Geometry check sheet. Reference: the model listing, model coordinates, mm. Face numbers are marked on the shaded views. A direction names the side the tool comes from. Give positions to 0.01 mm unless a question says otherwise; leave off trailing zeros. Order: outer loops, then holes, each group sorted by start corner. A loop starts at its lowest first (then second) coordinate and runs counter-clockwise, first axis right, second up. Notation, with made-up numbers: M 30.25,-10.5 L 82.25,-10.5 A15 ccw 82.25,9.5 Z; hole C 59,50.5 d2. An arc over 180 degrees is marked long. Answer as CSV lines item,"result". Start each with the question number.
Q1. Section check D-D, the plane x = 58.5. Record the boundary of the cut face in (y, z).
Q2. Thickness scan on line 1 (Y direction, x = 50, z = 13.45); line 2 (X direction, y = 160, z = 13.25); line 3 (Z direction, x = 55.5, y = 160.5). Record the ranges inside material, lowest first.
Q3. Section check C-C, the plane x = 50. Record the boundary of the cut face in (y, z), then the cut area to 3 significant figures.
Q4. Set-up check for the marked faces 1, 2, 3 and 4: record each of +Z, -Z, +X, -X, +Y, -Y from which the full face is reachable in a straight line by a thin tool's end or side.
Q5. Section check B-B, the plane y = 160. Record the boundary of the cut face in (x, z).
Q6. Section check A-A, the plane z = 13.55. Record the boundary of the cut face in (x, y), then the cut area to 3 significant figures.
Q7. Go/stop test with flat-tipped pins: pin 1 (0.8 mm diameter, centred on x = 46, z = 13.5, fed in from +Y); pin 2 (2.5 mm diameter, centred on x = 57, z = 13, fed in from -Y); pin 3 (0.9 mm diameter, centred on x = 61, z = 14, fed in from -Y). Record where each tip stops, or that it passes through.
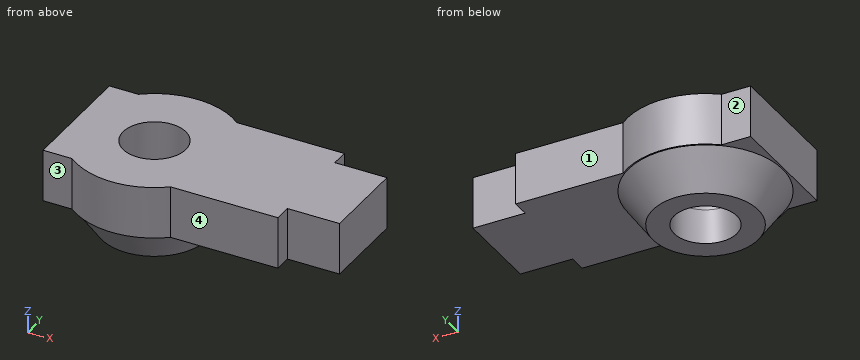
```python
from build123d import *

# Parameters (mm, degrees)
SKETCH164_R     = 1.8
PAD127002_DEPTH = 3


with BuildPart() as innerbearingrace:
    # Sketch165 → Revolution008 (revolve)
    with BuildSketch(Plane(origin=(50, 160, 10), x_dir=(1, 0, 0), z_dir=(0, -1, 0))):
        Polygon((4.423355, 2), (3.02294, 0), (1.8, 0), (1.8, 2), align=None)
    revolve(axis=Axis((50, 160, 10), (0, 0, 1)))


with BuildPart() as steeringcolumn_short:
    # Sketch164 → Pad127002 (new body)
    with BuildSketch(Plane(origin=(50, 160, 12), x_dir=(1, 0, 0), z_dir=(0, 0, 1))):
        with BuildLine():
            Line((9, 3.5), (2.828427, 3.5))
            ThreePointArc((2.828427, 3.5), (0, 4.5), (-2.828427, 3.5))
            Line((-2.828427, 3.5), (-4.5, 3.5))
            Line((-4.5, 3.5), (-4.5, -3.5))
            Line((-4.5, -3.5), (-2.828427, -3.5))
            ThreePointArc((-2.828427, -3.5), (0, -4.5), (2.828427, -3.5))
            Line((2.828427, -3.5), (9, -3.5))
            Line((9, -2.5), (9, -3.5))
            Line((12, -2.5), (9, -2.5))
            Line((12, 2.5), (12, -2.5))
            Line((9, 2.5), (12, 2.5))
            Line((9, 3.5), (9, 2.5))
        make_face()
        Circle(SKETCH164_R, mode=Mode.SUBTRACT)
    extrude(amount=PAD127002_DEPTH)

    # Fusion004020021: union InnerBearingRace
    add(innerbearingrace.part)


solid = steeringcolumn_short.part
```
Answer block:
1,outline,"M 156.5,12 L 163.5,12 L 163.5,15 L 156.5,15 Z"
2,line 1,"y = 155.5 to 158.2, 161.8 to 164.5"
2,line 2,"x = 45.5 to 48.2, 51.8 to 62"
2,line 3,"z = 12 to 15"
3,outline,"M 155.5,12 L 155.58,12 L 156.98,10 L 158.2,10 L 158.2,15 L 155.5,15 Z; M 161.8,10 L 163.02,10 L 164.42,12 L 164.5,12 L 164.5,15 L 161.8,15 Z"
3,area,"23.9 mm2"
4,face 1,"+Z, -Z, +X, +Y"
4,face 2,"+Z, -Z, -X, +Y"
4,face 3,"+Z, -Z, -X, -Y"
4,face 4,"+Z, -Z, +X, -Y"
5,outline,"M 45.5,12 L 45.58,12 L 46.98,10 L 48.2,10 L 48.2,15 L 45.5,15 Z; M 51.8,10 L 53.02,10 L 54.42,12 L 62,12 L 62,15 L 51.8,15 Z"
6,outline,"M 45.5,156.5 L 47.17,156.5 A4.5 ccw 52.83,156.5 L 59,156.5 L 59,157.5 L 62,157.5 L 62,162.5 L 59,162.5 L 59,163.5 L 52.83,163.5 A4.5 ccw 47.17,163.5 L 45.5,163.5 Z; hole C 50,160 d3.6"
6,area,"107 mm2"
7,pin 1,"stops at y = 163.5"
7,pin 2,"stops at y = 156.5"
7,pin 3,"stops at y = 157.5"
